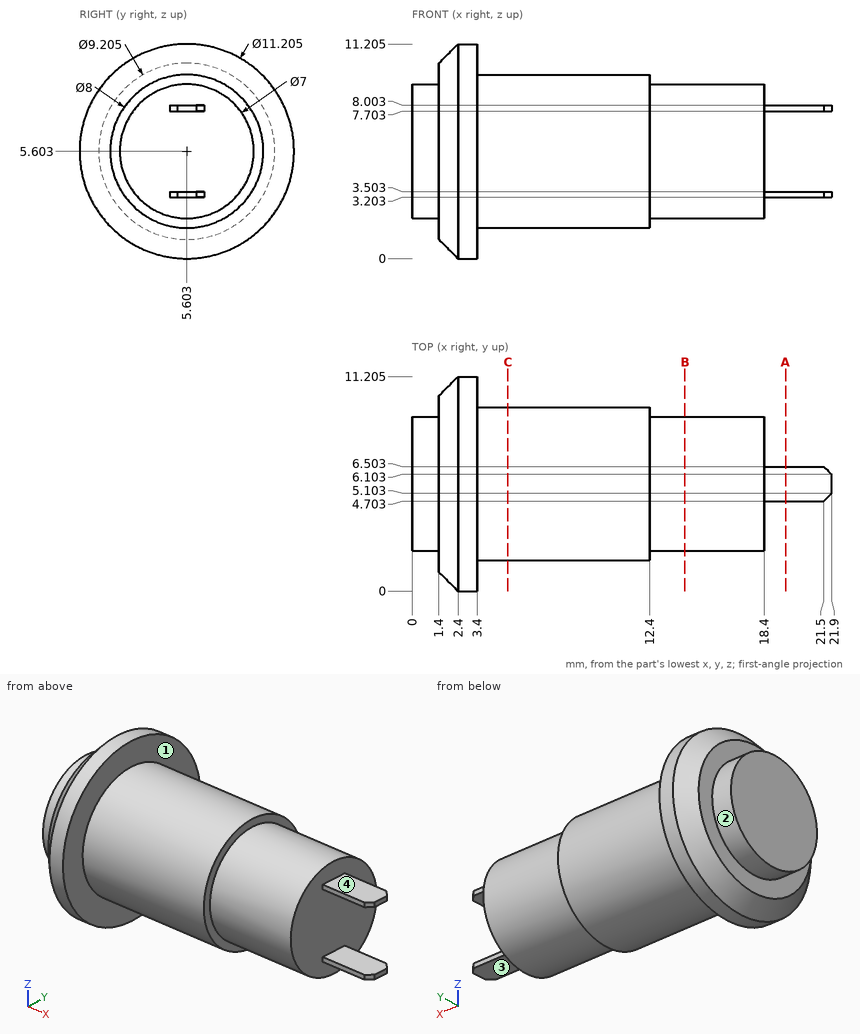
Part print with two shaded views. Sizes in mm from the minimum x, y, z corner. A direction names the side the tool comes from. Round coordinates to 2 decimals unless told otherwise and drop trailing zeros. Order: outer loops, then holes, each group sorted by start corner. A loop starts at its lowest first (then second) coordinate and runs counter-clockwise, first axis right, second up. Notation, with made-up numbers: (19.5, -23) - (58.5, -23) arc R24 cw to (58.5, 6) - close; hole circle Ø10 at (16.5, -26.5). An arc over 180 degrees is marked (long way). Answer in a Markdown table with one row per item. Add a question column.
(1) Probe L1, parallel to X at y = 3.75, z = 9; L2, parallel to X at y = 6.75, z = 8.5; L3, parallel to Y at x = 9.25, z = 2 (1 decimal). List the from-to ranges inside material, lowest first. Write a range as [from, to].
(2) Drop flat-ended pins along their axis: pin 1 Ø1.4 at (x, y) = (20.5, 5.5) entering from +Z; pin 2 Ø2.5 at (y, z) = (7.5, 6.5) entering from +X; pin 3 Ø4 at (x, y) = (3, 8.5) entering from -Z. Give the stop position or say it passes through.
(3) Band-saw the part on C-C on x = 5. List the corners of the cut face in (y, z).
(4) 3-axis set-ups, long thin cutter, end or side, ignore diameter. For the marked faces 1, 2, 3 and 4: which of +Z, -Z, +X, -X, +Y, -Y reach the whole face in a straight line?
(5) Band-saw the part on B-B on x = 14.25. List the corners of the cut face in (y, z).
(6) Band-saw the part on A-A on x = 19.5. List the corners of the cut face in (y, z).
Data:
| question | item | result |
|---|---|---|
| 1 | L1 | x = [1.4, 12.4] |
| 1 | L2 | x = [0, 18.4] |
| 1 | L3 | y = [3.9, 7.3] |
| 2 | pin 1 | stops at z = 8 |
| 2 | pin 2 | stops at x = 18.4 |
| 2 | pin 3 | stops at z = 0.07 |
| 3 | outline | circle Ø8 at (5.6, 5.6) |
| 4 | face 1 | +X |
| 4 | face 2 | -X |
| 4 | face 3 | -Z, +X, +Y, -Y |
| 4 | face 4 | +Z, +X, +Y, -Y |
| 5 | outline | circle Ø7 at (5.6, 5.6) |
| 6 | outline | (4.7, 3.2) - (6.5, 3.2) - (6.5, 3.5) - (4.7, 3.5) - close; (4.7, 7.7) - (6.5, 7.7) - (6.5, 8) - (4.7, 8) - close |
